```python
from build123d import *

# Parameters (mm, degrees)
CHAMFER_1_SIZE = 0.5


with BuildPart() as part:
    # 草图1 → 旋转1 (revolve)
    with BuildSketch(Plane(origin=(0, 0, 0), x_dir=(1, 0, 0), z_dir=(0, 1, 0))):
        Polygon((-8.630363036, 0), (-8.630363036, 5), (-3.630363036, 5), (-3.630363036, 6), (48.369636964, 6), (48.369636964, 5), (66.369636964, 5), (66.369636964, 0), align=None)
    revolve(axis=Axis((66.369636964, 0, 0), (-1, 0, 0)))

    # 倒角1
    chamfer_1_edges = [part.edges().sort_by_distance(p)[0] for p in [
        (66.369636964, 0, 5),
        (-8.630363036, 0, 5),
    ]]
    chamfer(chamfer_1_edges, length=CHAMFER_1_SIZE)


solid = part.part
```
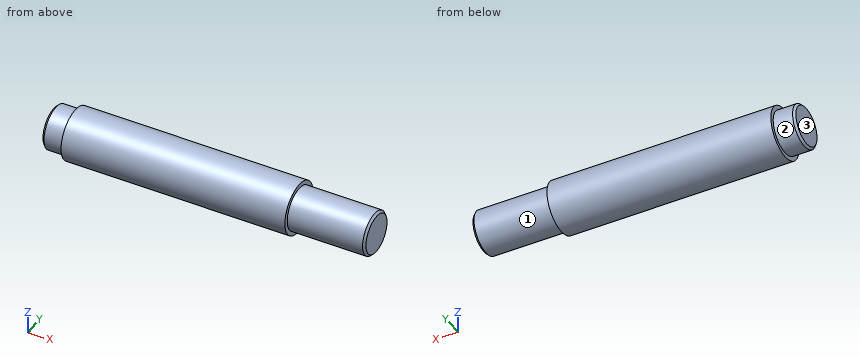
Verification items for the finished model (mm, model axes). Face numbers are marked on the shaded views. A direction names the side the tool comes from. Coordinates: 2 decimals unless noted, no trailing zeros. Write each loop counter-clockwise with the first axis right and the second up, starting at its lowest first coordinate (ties: lowest second). Pieces come first, ordered by that corner, then holes. Notation, with made-up numbers: (-18.75, 75) - (-12.75, 75) arc R18 cw to (-12.75, 110) - close; hole circle Ø8 at (-32, 18). An arc over 180 degrees is marked (long way). Write item = value, one per line.
Q1. Cross-section at C-C (x = 62). Enter the section's corners in (y, z).
Answer:
outline = circle Ø10 at (0, 0)
Q2. Access from +Z, -Z, +X, -X, +Y, -Y to the whole of each face (thin tool, end or side, straight path). Record for the marked faces 1, 2 and 3.
Answer:
face_1 = +X
face_2 = -X
face_3 = +Z, -Z, -X, +Y, -Y
Q3. Cross-section at A-A (y = 0). Enter the section's corners in (x, z), plus the area to 4 significant figures.
Answer:
outline = (-8.63, -4.5) - (-8.13, -5) - (-3.63, -5) - (-3.63, -6) - (48.37, -6) - (48.37, -5) - (65.87, -5) - (66.37, -4.5) - (66.37, 4.5) - (65.87, 5) - (48.37, 5) - (48.37, 6) - (-3.63, 6) - (-3.63, 5) - (-8.13, 5) - (-8.63, 4.5) - close
area = 853.5 mm²
Q4. Go/stop test with flat-tipped pins: pin 1 Ø4 at (x, y) = (53.5, -4.5) entering from +Z; pin 2 Ø1.5 at (x, z) = (46, -2.5) entering from +Y; pin 3 Ø1 at (y, z) = (4, -4.5) entering from +X. Record where each tip stops, or that it passes through.
Answer:
pin_1 = 4.33
pin_2 = 5.74
pin_3 = 48.37
Q5. Material ranges on L1, parallel to X at y = 4.5, z = 3.5; L2, parallel to Y at x = -4, z = 0.25, recorded low to high. Write a range as from..to.
Answer:
L1 = -3.63..48.37
L2 = -4.99..4.99
Q6. Cross-section at D-D (x = 16.5). Enter the section's corners in (y, z), plus the area to 3 significant figures.
Answer:
outline = circle Ø12 at (0, 0)
area = 113 mm²
